Read the model definition and answer for the solid it produces. Units are mm, in the model's axes. A direction names the side the tool comes from. Give positions to 0.01 mm unless a question says otherwise; leave off trailing zeros. Write each loop counter-clockwise with the first axis right and the second up, starting at its lowest first coordinate (ties: lowest second). Pieces come first, ordered by that corner, then holes. Notation, with made-up numbers: M -18,44 L -6,44 A6 cw -6,53 Z; hole C -39,-23 d1. An arc over 180 degrees is marked long. Use a Markdown table: item, result. Add a question column.
Item 1: Consider probe 1 along Y at (x, z) = (10.65, 0); probe 2 along X at (y, z) = (1, 8.5) (3 decimals); probe 3 along Y at (x, z) = (3.25, 0). Determine where each line is inside the solid, lowest interval first. Write a range as [from, to].
Item 2: The mould has two halves that part along Z. Classify faces 6 (the cylindrical face through (11.94, -37.95, 0.23)), 7 (the flat face through (3.937, 25.6, 23)), 8 (the cylindrical face through (2.32, -27.695, 21.236)): pulls with the +Z half, pulls with the -Z half, needs draft (parallel to the pull), parting line crosses it, or undercut.
Item 3: Given P1, Ø2, axis at x = 6, z = 12, coming from the +Y side; P2, Ø4.5, axis at y = -28.06, z = 28.06, coming from the -X side (3 decimals); P3, Ø2, axis at y = -39.69, z = 0, coming from the +X side; P4, Ø5, axis at x = 3.5, z = -24.5, coming from the +Y side, each flat-ended and moving along its own axis, determine where each tip first touches the part or whether it passes through.
Item 4: A cutting plane is placed at A-A on z = 0. Count the separate pieces of the cut face and the enclosed holes in it, then the cut area to 3 significant figures.
Item 5: For faces 1 (the flat face through (9.525, 6, -35)), 2 (the flat face through (9.525, -4.2, -4.2)), 3 (the flat face through (0, -7, 0)), 4 (the cylindrical face through (11.94, -29.774, 28.443)), 5 (the cylindrical face through (5.155, -7.296, 32.855)), determine the directions among +Z, -Z, +X, -X, +Y, -Y from which every point of the face is accessible in a straight line to the end or side of a thin tool.
Item 6: A cutting plane is placed at B-B on x = 12.5. Determine the outline of the cut face in (y, z) (1 decimal).
from build123d import *

# Parameters (mm, degrees)
M3_CLEARANCE_HOLE1_D                     = 3.5052
M3_CLEARANCE_HOLE1_DEPTH                 = 4.7625
CBORE_FOR_M10_HEX_HEAD_BOLT1_D           = 11.1125
CBORE_FOR_M10_HEX_HEAD_BOLT1_DEPTH       = 14.2875
CBORE_FOR_M10_HEX_HEAD_BOLT1_CBORE_D     = 19.685
CBORE_FOR_M10_HEX_HEAD_BOLT1_CBORE_DEPTH = 4.7625
CHAMFER1_SIZE                            = 0.381
CHAMFER2_SIZE                            = 0.7874
FILLET1_R                                = 0.127
FILLET2_R                                = 0.381


with BuildPart() as part:
    # Sketch1 → Revolve1 (revolve)
    with BuildSketch(Plane(origin=(0, 0, 0), x_dir=(-1, 0, 0), z_dir=(0, 0, -1))):
        Polygon((-14.2875, 42.7355), (-14.2875, 0), (0, 0), (0, 34.8996), (-3.937, 34.8996), (-3.937, 33.655), (-6.35, 33.655), (-6.35, 34.8996), (-9.525, 34.8996), (-9.525, 42.7355), align=None)
    revolve(axis=Axis((14.2875, 0, 0), (-1, 0, 0)))

    # M3 Clearance Hole1
    with Locations(Plane.ZY.offset(-9.525)):
        with Locations((28.063300378, -28.063300378), (-28.063300378, 28.063300378), (39.6875, 0), (-39.6875, 0), (0, -39.6875), (0, 39.6875)):
            Hole(M3_CLEARANCE_HOLE1_D / 2, depth=M3_CLEARANCE_HOLE1_DEPTH)

    # CBORE for M10 Hex Head Bolt1
    with Locations(Plane(origin=(14.2875, 0, 0), x_dir=(0, 0, -1), z_dir=(1, 0, 0))):
        with Locations((0, 0)):
            CounterBoreHole(CBORE_FOR_M10_HEX_HEAD_BOLT1_D / 2, CBORE_FOR_M10_HEX_HEAD_BOLT1_CBORE_D / 2, CBORE_FOR_M10_HEX_HEAD_BOLT1_CBORE_DEPTH, depth=CBORE_FOR_M10_HEX_HEAD_BOLT1_DEPTH)

    # Chamfer1
    chamfer1_edges = [part.edges().sort_by_distance(p)[0] for p in [
        (14.2875, -42.7355, 0),
        (9.525, -42.7355, 0),
    ]]
    chamfer(chamfer1_edges, length=CHAMFER1_SIZE)

    # Chamfer2
    chamfer2_edges = [part.edges().sort_by_distance(p)[0] for p in [
        (0, -34.8996, 0),
    ]]
    chamfer(chamfer2_edges, length=CHAMFER2_SIZE)

    # Fillet1
    fillet1_edges = [part.edges().sort_by_distance(p)[0] for p in [
        (6.35, -34.8996, 0),
        (3.937, -34.8996, 0),
    ]]
    fillet(fillet1_edges, radius=FILLET1_R)

    # Fillet2
    fillet2_edges = [part.edges().sort_by_distance(p)[0] for p in [
        (6.35, -33.655, 0),
        (3.937, -33.655, 0),
    ]]
    fillet(fillet2_edges, radius=FILLET2_R)


solid = part.part
Filled in:
| question | item | result |
|---|---|---|
| 1 | probe 1 | [-42.74, -41.44], [-37.93, -9.84], [9.84, 37.93], [41.44, 42.74] |
| 1 | probe 2 | [0, 9.525] |
| 1 | probe 3 | [-34.9, -5.56], [5.56, 34.9] |
| 2 | face 6 | undercut |
| 2 | face 7 | needs draft |
| 2 | face 8 | parting line crosses it |
| 3 | P1 | y = 33.08 |
| 3 | P2 | x = 9.525 |
| 3 | P3 | through |
| 3 | P4 | y = 27.09 |
| 4 | separate pieces | 4 |
| 4 | enclosed holes | 0 |
| 4 | area | 832 mm² |
| 5 | face 1 | -X |
| 5 | face 2 | +X |
| 5 | face 3 | +Z, -Z, -X, +Y, -Y |
| 5 | face 4 | +X, -X |
| 5 | face 5 | none |
| 6 | outline | C 0,0 d85.5; hole C -39.7,0 d3.5; hole C -28.1,28.1 d3.5; hole C 0,0 d19.7; hole C 0,-39.7 d3.5; hole C 0,39.7 d3.5; hole C 28.1,-28.1 d3.5; hole C 39.7,0 d3.5 |
